from build123d import *
from OCP.BRepFilletAPI import BRepFilletAPI_MakeChamfer

# Parameters (mm, degrees)
SKETCH1_W           = 50
SKETCH1_H           = 100
BOSS_EXTRUDE1_DEPTH = 4
FILLET1_R           = 3
FILLET2_R           = 3
SKETCH2_R           = 4.75
BOSS_EXTRUDE2_DEPTH = 10
CHAMFER1_SIZE       = 3
CHAMFER1_SIZE2      = 1.212078678


with BuildPart() as part:
    # Sketch1 → Boss-Extrude1 (new body)
    with BuildSketch(Plane.XY):
        Rectangle(SKETCH1_W, SKETCH1_H)
    extrude(amount=BOSS_EXTRUDE1_DEPTH)

    # Fillet1
    fillet1_edges = [part.edges().sort_by_distance(p)[0] for p in [
        (-25, 0, 4),
        (0, -50, 4),
        (25, 0, 4),
        (0, 50, 4),
    ]]
    fillet(fillet1_edges, radius=FILLET1_R)

    # Fillet2
    # the kernel refuses this fillet: 3 mm, written as the material it takes off along each edge
    with BuildSketch(Plane(origin=(-22, 47, 1), x_dir=(0, 1, 0), z_dir=(-1, 0, 0))) as fillet2_piece_1_section:
        Polygon((0, 0), (FILLET2_R, 0), (FILLET2_R, -FILLET2_R), (0, -FILLET2_R), align=None)
    fillet2_piece_1 = extrude(amount=FILLET2_R, mode=Mode.PRIVATE)
    fillet2_piece_1 = fillet2_piece_1 - Plane(origin=(-22, 47, 1), x_dir=(0, -0.7071067811865475, -0.7071067811865475), z_dir=(-1, 0, 0)) * Sphere(FILLET2_R, mode=Mode.PRIVATE)
    add(fillet2_piece_1, mode=Mode.SUBTRACT)
    with BuildSketch(Plane(origin=(22, 47, 1), x_dir=(0, 1, 0), z_dir=(1, 0, 0))) as fillet2_piece_2_section:
        Polygon((0, 0), (FILLET2_R, 0), (FILLET2_R, FILLET2_R), (0, FILLET2_R), align=None)
    fillet2_piece_2 = extrude(amount=FILLET2_R, mode=Mode.PRIVATE)
    fillet2_piece_2 = fillet2_piece_2 - Plane(origin=(22, 47, 1), x_dir=(0, -0.7071067811865475, -0.7071067811865475), z_dir=(1, 0, 0)) * Sphere(FILLET2_R, mode=Mode.PRIVATE)
    add(fillet2_piece_2, mode=Mode.SUBTRACT)
    with BuildSketch(Plane(origin=(-22, -47, 1), x_dir=(-1, 0, 0), z_dir=(0, -1, 0))) as fillet2_piece_3_section:
        Polygon((0, 0), (FILLET2_R, 0), (FILLET2_R, -FILLET2_R), (0, -FILLET2_R), align=None)
    fillet2_piece_3 = extrude(amount=FILLET2_R, mode=Mode.PRIVATE)
    fillet2_piece_3 = fillet2_piece_3 - Plane(origin=(-22, -47, 1), x_dir=(0.7071067811865475, 0, -0.7071067811865475), z_dir=(0, -1, 0)) * Sphere(FILLET2_R, mode=Mode.PRIVATE)
    add(fillet2_piece_3, mode=Mode.SUBTRACT)
    with BuildSketch(Plane(origin=(22, -47, 1), x_dir=(1, 0, 0), z_dir=(0, -1, 0))) as fillet2_piece_4_section:
        Polygon((0, 0), (FILLET2_R, 0), (FILLET2_R, FILLET2_R), (0, FILLET2_R), align=None)
    fillet2_piece_4 = extrude(amount=FILLET2_R, mode=Mode.PRIVATE)
    fillet2_piece_4 = fillet2_piece_4 - Plane(origin=(22, -47, 1), x_dir=(-0.7071067811865475, 0, -0.7071067811865475), z_dir=(0, -1, 0)) * Sphere(FILLET2_R, mode=Mode.PRIVATE)
    add(fillet2_piece_4, mode=Mode.SUBTRACT)
    with BuildSketch(Plane(origin=(25, -50, -7.5), x_dir=(-1, 0, 0), z_dir=(0, 0, 1)), Plane(origin=(25, 50, -7.5), x_dir=(0, -1, 0), z_dir=(0, 0, 1))) as fillet2_piece_5:
        with BuildLine():
            CenterArc((FILLET2_R, -FILLET2_R), FILLET2_R, 90, 90)
            Line((0, -FILLET2_R), (0, 0))
            Line((0, 0), (FILLET2_R, 0))
        make_face()
    extrude(amount=8.5, mode=Mode.SUBTRACT)
    with BuildSketch(Plane(origin=(-25, -50, -7.5), x_dir=(1, 0, 0), z_dir=(0, 0, 1)), Plane(origin=(-25, 50, -7.5), x_dir=(0, -1, 0), z_dir=(0, 0, 1))) as fillet2_piece_6:
        with BuildLine():
            CenterArc((FILLET2_R, FILLET2_R), FILLET2_R, 180, 90)
            Line((0, FILLET2_R), (0, 0))
            Line((0, 0), (FILLET2_R, 0))
        make_face()
    extrude(amount=8.5, mode=Mode.SUBTRACT)

    # Sketch2 → Boss-Extrude2 (add)
    with BuildSketch(Plane(origin=(0, 0, 0), x_dir=(-1, 0, 0), z_dir=(0, 0, -1))):
        with Locations((0, 25)):
            Circle(SKETCH2_R)
        with Locations((0, -25)):
            Circle(SKETCH2_R)
    extrude(amount=BOSS_EXTRUDE2_DEPTH)

    # Chamfer1: one chamfer whose edges measure the first distance from different faces: ONE call of the kernel's chamfer builder (chamfer() names one face for all edges)
    chamfer1_edges_1 = [part.edges().sort_by_distance(p)[0] for p in [
        (4.75, 25, -10),
    ]]
    chamfer1_side_1 = [part.faces().sort_by_distance(p)[0] for p in [
        (4.75, 25, -5),
    ]]
    chamfer1_edges_2 = [part.edges().sort_by_distance(p)[0] for p in [
        (4.75, -25, -10),
    ]]
    chamfer1_side_2 = [part.faces().sort_by_distance(p)[0] for p in [
        (4.75, -25, -5),
    ]]
    chamfer1 = BRepFilletAPI_MakeChamfer(part.part.solid().wrapped)
    for e in chamfer1_edges_1:
        chamfer1.Add(CHAMFER1_SIZE, CHAMFER1_SIZE2, e.wrapped, chamfer1_side_1[0].wrapped)  # the first distance lies on this face
    for e in chamfer1_edges_2:
        chamfer1.Add(CHAMFER1_SIZE, CHAMFER1_SIZE2, e.wrapped, chamfer1_side_2[0].wrapped)  # the first distance lies on this face
    add(Compound.cast(chamfer1.Shape()), mode=Mode.REPLACE)


solid = part.part
Here's how the part is built. I have some questions about the finished solid (model axes, mm). A direction names the side the tool comes from. Coordinates: 2 decimals unless noted, no trailing zeros. Loops run counter-clockwise (first coordinate to the right, second up) from the corner with the lowest first, then second, coordinate; pieces in that order, holes last.
1. For P1, Ø1, axis at x = 10.5, y = 2, coming from the -Z side, with a flat end and sliding along its axis, tell me the tip position at first contact or that it passes through.
2. I need wall thicknesses on L1, parallel to Z at x = -4, y = -20.5; L2, parallel to Y at x = 3, z = -5.25; L3, parallel to Y at x = -22, z = 1.25. Which ranges of each line are inside material? Lowest first, please.
3. Imagine slicing it at D-D, the plane x = 13. Please give me the cut outline in (y, z), and give its area (3 significant figures).
4. Imagine slicing it at A-A, the plane x = 0. Please give me the cut outline in (y, z), and give its area (3 significant figures).
5. Imagine slicing it at C-C, the plane z = -5. Please give me the cut outline in (x, y).
6. If we mould it in two halves opening along Y, with no side actions, what happens to faces 3 (the cylindrical face through (0.31, 49.14, 3.1)), 4 (the flat face through (0, 25, -10)), 5 (the cylindrical face through (0.62, -20.29, -3.45))? For each: pulls with the +Y half, pulls with the -Y half, needs draft (parallel to the pull), parting line crosses it, or undercut.
7. Imagine slicing it at B-B, the plane y = -25. Please give me the cut outline in (x, z), and give its area (3 significant figures).
8. For faces 1 (the flat face through (0, 1, 4)), 2 (the cylindrical face through (0.62, 29.71, -3.45)), which set-ups out of +Z, -Z, +X, -X, +Y, -Y let a thin tool reach every point of the face, with its end or its side?
Taken from the geometry:
1. P1: stops at z = 0
2. L1: z = 0 to 4
2. L2: y = -28.68 to -21.32, 21.32 to 28.68
2. L3: y = -49.99 to 49.99
3. outline: (-50, 0) - (50, 0) - (50, 1) arc R3 ccw to (47, 4) - (-47, 4) arc R3 ccw to (-50, 1) - close
3. area: 396 mm2
4. outline: (-50, 0) - (-29.75, 0) - (-29.75, -7) - (-28.54, -10) - (-21.46, -10) - (-20.25, -7) - (-20.25, 0) - (20.25, 0) - (20.25, -7) - (21.46, -10) - (28.54, -10) - (29.75, -7) - (29.75, 0) - (50, 0) - (50, 1) arc R3 ccw to (47, 4) - (-47, 4) arc R3 ccw to (-50, 1) - close
4. area: 579 mm2
5. outline: circle Ø9.5 at (0, -25); circle Ø9.5 at (0, 25)
6. face 3: pulls with the +Y half
6. face 4: needs draft
6. face 5: undercut
7. outline: (-25, 0) - (-4.75, 0) - (-4.75, -7) - (-3.54, -10) - (3.54, -10) - (4.75, -7) - (4.75, 0) - (25, 0) - (25, 1) arc R3 ccw to (22, 4) - (-22, 4) arc R3 ccw to (-25, 1) - close
7. area: 288 mm2
8. face 1: +Z, +X, -X, +Y, -Y
8. face 2: -Z
